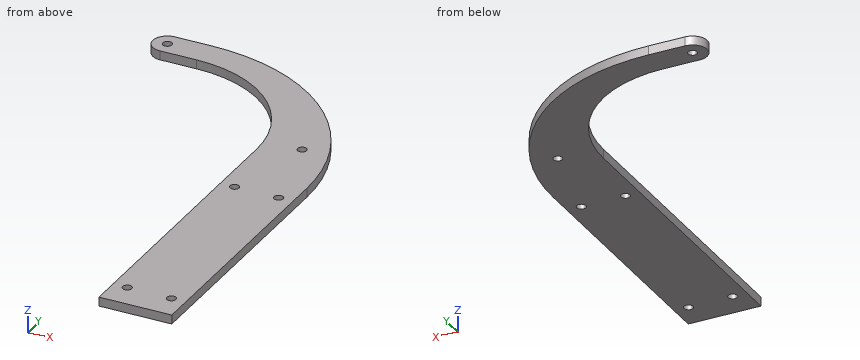
from build123d import *

# Parameters (mm, degrees)
SKETCH1_R           = 3.175
BOSS_EXTRUDE1_DEPTH = 6.35


with BuildPart() as part:
    # Sketch1 → Boss-Extrude1 (new body)
    with BuildSketch(Plane.XY):
        with BuildLine():
            Line((0, 10.16), (25.4, 10.16))
            ThreePointArc((25.4, 10.16), (122.061496988, -29.878503012), (162.1, -126.54))
            Line((162.1, -126.54), (162.1, -310.482187261))
            Line((162.1, -310.482187261), (111.3, -310.482187261))
            Line((111.3, -310.482187261), (111.3, -96.06))
            ThreePointArc((111.3, -96.06), (86.140472504, -35.319527496), (25.4, -10.16))
            Line((25.4, -10.16), (0, -10.16))
            ThreePointArc((0, -10.16), (-10.16, 0), (0, 10.16))
        make_face()
        Circle(SKETCH1_R, mode=Mode.SUBTRACT)
        with Locations((136.7, -83.36)):
            Circle(SKETCH1_R, mode=Mode.SUBTRACT)
        with Locations((121.3, -291.432187261)):
            Circle(SKETCH1_R, mode=Mode.SUBTRACT)
        with Locations((152.1, -291.432187261)):
            Circle(SKETCH1_R, mode=Mode.SUBTRACT)
        with Locations((121.3, -145.382187261)):
            Circle(SKETCH1_R, mode=Mode.SUBTRACT)
        with Locations((152.1, -145.382187261)):
            Circle(SKETCH1_R, mode=Mode.SUBTRACT)
    extrude(amount=BOSS_EXTRUDE1_DEPTH)


solid = part.part
For this review, take the finished solid that the model builds, in its own axes (mm). Round coordinates to 2 decimals unless told otherwise and drop trailing zeros. Loops run counter-clockwise (first coordinate to the right, second up) from the corner with the lowest first, then second, coordinate; pieces in that order, holes last. Notation, with made-up numbers: (3, 43) - (40, 43) arc R16 ccw to (40, 68) - close; hole circle Ø8 at (77.5, 79.5). An arc over 180 degrees is marked (long way). Put each result on its own line as item: value. Start each with the question number.
1. Consider section C-C on z = 4.25. State the section outline as (x, y) points (3 decimals).
2. For probe 1 along X at (y, z) = (-294, 2); probe 2 along X at (y, z) = (-263.5, 1.25); probe 3 along Y at (x, z) = (121.3, 2.25), list the stretches that pass through material, from the lowest coordinate up. Write a range as [from, to].
3. Consider section A-A on x = 121.3. State the section outline as (y, z) points, plus the area to 3 significant figures.
4. Consider section B-B on y = -83.36. State the section outline as (x, z) points (3 decimals).
5. Insertion check: P1, Ø3, axis at x = 15, z = 3, coming from the -Y side. The pin has a flat end and moves straight along its axis. Give the tip position at first contact, or say it passes through.
6. Consider section D-D on y = -160.5. State the section outline as (x, z) points, plus the area to 3 significant figures.
Result sheet:
1. outline: (0, -10.16) - (25.4, -10.16) arc R85.9 cw to (111.3, -96.06) - (111.3, -310.482) - (162.1, -310.482) - (162.1, -126.54) arc R136.7 ccw to (25.4, 10.16) - (0, 10.16) arc R10.16 ccw to start; hole circle Ø6.35 at (0, 0); hole circle Ø6.35 at (121.3, -291.432); hole circle Ø6.35 at (121.3, -145.382); hole circle Ø6.35 at (136.7, -83.36); hole circle Ø6.35 at (152.1, -291.432); hole circle Ø6.35 at (152.1, -145.382)
2. probe 1: [111.3, 119.43], [123.17, 150.23], [153.97, 162.1]
2. probe 2: [111.3, 162.1]
2. probe 3: [-310.48, -294.61], [-288.26, -148.56], [-142.21, -29.12]
3. outline: (-310.48, 0) - (-294.61, 0) - (-294.61, 6.35) - (-310.48, 6.35) - close; (-288.26, 0) - (-148.56, 0) - (-148.56, 6.35) - (-288.26, 6.35) - close; (-142.21, 0) - (-29.12, 0) - (-29.12, 6.35) - (-142.21, 6.35) - close
3. area: 1,710 mm^2
4. outline: (110.356, 0) - (133.525, 0) - (133.525, 6.35) - (110.356, 6.35) - close; (139.875, 0) - (155.101, 0) - (155.101, 6.35) - (139.875, 6.35) - close
5. P1: y = -10.16
6. outline: (111.3, 0) - (162.1, 0) - (162.1, 6.35) - (111.3, 6.35) - close
6. area: 323 mm^2
